Here's how the part is built. I have some questions about the finished solid (model axes, mm). A direction names the side the tool comes from. Round coordinates to 2 decimals unless told otherwise and drop trailing zeros. Order: outer loops, then holes, each group sorted by start corner. A loop starts at its lowest first (then second) coordinate and runs counter-clockwise, first axis right, second up. Notation, with made-up numbers: (30, -14.5) - (73, -14.5) arc R31 ccw to (73, 18.5) - close; hole circle Ø7 at (52, -12). An arc over 180 degrees is marked (long way). One line per item, written item: value.
from build123d import *

# Parameters (mm, degrees)
F0_R      = 37
F1_DEPTH  = 120
F2_R      = 30
F3_DEPTH  = 80
F5_D      = 12
F5_DEPTH  = 22
F5_TIP    = 3.6051637142
F9_D      = 5.5
F9_DEPTH  = 15
F9_TIP    = 1.6523667023
F11_D     = 3.3
F11_DEPTH = 15
F11_TIP   = 0.9914200214


with BuildPart() as f1:
    # F0 (on Top) → F1 (new body)
    with BuildSketch(Plane.XY):
        Circle(F0_R)
    extrude(amount=F1_DEPTH)

    # F2 (on face) → F3 (cut)
    with BuildSketch(Plane(origin=(0, 0, 0), x_dir=(1, 0, 0), z_dir=(0, 0, -1))):
        Circle(F2_R)
    extrude(amount=-F3_DEPTH, mode=Mode.SUBTRACT)

    # F5
    with Locations(Plane.XY.offset(120)):
        with Locations((0, 0)):
            Hole(F5_D / 2, depth=F5_DEPTH)
            with Locations((0, 0, -(F5_DEPTH + F5_TIP / 2))):  # 118° drill point
                Cone(0, F5_D / 2, F5_TIP, mode=Mode.SUBTRACT)

    # F6 (on Front) → F7 (revolve, cut)
    with BuildSketch(Plane.XZ):
        with BuildLine():
            Line((-8.50013727, 120), (-11.5, 120))
            Line((-11.5, 120), (-11.5, 118.9797073603))
            ThreePointArc((-11.5, 118.9797073603), (-9.989853448, 117.4797416782), (-8.50013727, 119))
            Line((-8.50013727, 119), (-8.50013727, 120))
        make_face()
    revolve(axis=Axis((0, 0, 55.1168825477), (0, 0, -1)), mode=Mode.SUBTRACT)

    # F9
    with Locations(Plane.XY.offset(120)):
        with Locations((-25, 0), (0, 25), (25, 0), (0, -25)):
            Hole(F9_D / 2, depth=F9_DEPTH)
            with Locations((0, 0, -(F9_DEPTH + F9_TIP / 2))):  # 118° drill point
                Cone(0, F9_D / 2, F9_TIP, mode=Mode.SUBTRACT)

    # F11
    with Locations(Plane(origin=(0, 0, 0), x_dir=(1, 0, 0), z_dir=(0, 0, -1))):
        with Locations((-33.5, 0), (0, 33.5), (33.5, 0), (0, -33.5)):
            Hole(F11_D / 2, depth=F11_DEPTH)
            with Locations((0, 0, -(F11_DEPTH + F11_TIP / 2))):  # 118° drill point
                Cone(0, F11_D / 2, F11_TIP, mode=Mode.SUBTRACT)


solid = f1.part
Q1. If we section it at A-A, the plane z = 20: Please give me the cut outline in (x, y), then the cut area to 3 significant figures.
Results list:
outline: circle Ø74 at (0, 0); hole circle Ø60 at (0, 0)
area: 1,470 mm²
Q2. We'd pull the mould along Y, two halves only. Please class faces 1 (the flat face through (8, 9, 120)), 2 (the cylindrical face through (-22.253, 0.121, 112.395)): released by +Y, released by -Y, zero draft, split by the parting line, or undercut.
Results list:
face 1: zero draft
face 2: undercut
Q3. Will these pins go through, and if not, where does the flat tip stop? pin 1 (9 mm diameter, centred on x = -25, y = 0, fed in from +Z); pin 2 (5 mm diameter, centred on x = 25, y = 0, fed in from +Z); pin 3 (5 mm diameter, centred on x = -12, z = 67, fed in from -Y); pin 4 (2 mm diameter, centred on x = -23.5, y = -1, fed in from -Z).
Results list:
pin 1: z = 120
pin 2: z = 104.85
pin 3: y = -35.76
pin 4: z = 80
Q4. Which directions (+Z, -Z, +X, -X, +Y, -Y) give clear straight access to the entire face, cutting with the end or side of a thin tool? Please do faces 3 (the cylindrical face through (27.747, 0.121, 112.395)), 4 (the cylindrical face through (0.215, 31.864, 7.605)).
Results list:
face 3: +Z
face 4: -Z
Q5. If we section it at B-B, the plane z = 110: Please give me the cut outline in (x, y), then the cut area to 3 significant figures.
Results list:
outline: circle Ø74 at (0, 0); hole circle Ø5.5 at (-25, 0); hole circle Ø12 at (0, 0); hole circle Ø5.5 at (0, -25); hole circle Ø5.5 at (0, 25); hole circle Ø5.5 at (25, 0)
area: 4,090 mm²
Q6. If I drill on line 1 along Z through (x, y) = (-23.5, -17); line 2 along X through (y, z) = (-25, 112.5); line 3 along Y through (x, z) = (-27, 31), over which ranges is the centre line in solid material (lowest first)?
Results list:
line 1: 80 to 120
line 2: -27.28 to -2.75, 2.75 to 27.28
line 3: -25.3 to -13.08, 13.08 to 25.3
Q7. If we section it at C-C, the plane x = 13: Please give me the cut outline in (y, z).
Results list:
outline: (-34.64, 0) - (-27.04, 0) - (-27.04, 80) - (27.04, 80) - (27.04, 0) - (34.64, 0) - (34.64, 120) - (-34.64, 120) - close
Q8. If we section it at D-D, the plane y = 20: Please give me the cut outline in (x, z), then the cut area to 3 significant figures.
Results list:
outline: (-31.13, 0) - (-22.36, 0) - (-22.36, 80) - (22.36, 80) - (22.36, 0) - (31.13, 0) - (31.13, 120) - (-31.13, 120) - close
area: 3,890 mm²
